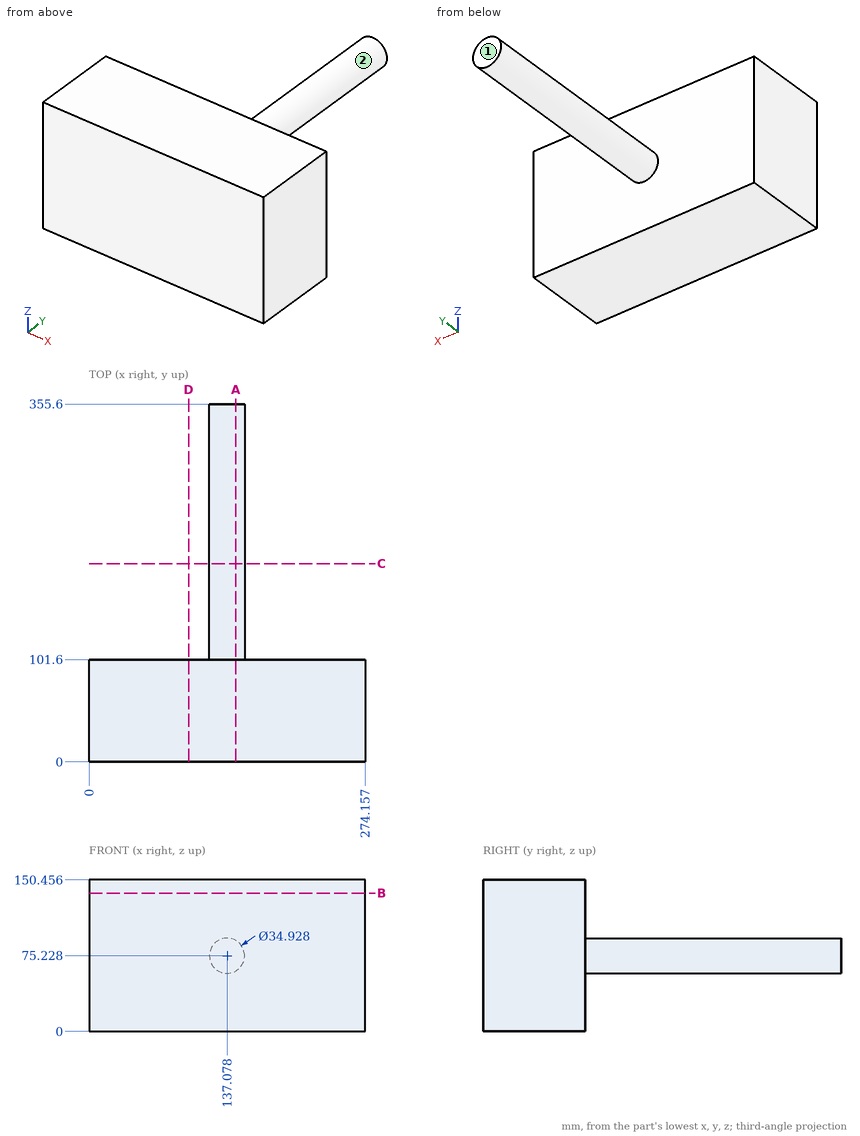
Print and shaded views of the part. All mm, measured from the part's lowest x, y and z. A direction names the side the tool comes from. Give positions to 0.01 mm unless a question says otherwise; leave off trailing zeros. Write each loop counter-clockwise with the first axis right and the second up, starting at its lowest first coordinate (ties: lowest second). Pieces come first, ordered by that corner, then holes. Notation, with made-up numbers: (43, 30) -> (72, 30) arc R16 ccw to (72, 50) -> close; hole circle Ø5 at (30, 46.5). An arc over 180 degrees is marked (long way). Use CSV: the item, a comma, the result in double quotes. Start each with the question number.
1) Cut at D-D on x = 99. List the corners of the cut face in (y, z) (1 decimal), plus the area to 3 significant figures.
2) Pin check, flat tips, straight feed: P1, Ø8, axis at y = 221.5, z = 93, coming from the -X side; P2, Ø5, axis at y = 204.5, z = 76, coming from the -X side (1 decimal). Stop position of each tip, or through.
3) Cut at B-B on z = 137.5. List the corners of the cut face in (x, y), plus the area to 3 significant figures.
4) Tool access for the marked faces 1 and 2: list every direction of +Z, -Z, +X, -X, +Y, -Y with a clear straight run to the whole face (end or side of a thin tool).
5) Drill centre lines: L1, parallel to Y at x = 113.5, z = 42.5; L2, parallel to Z at x = 143, y = 123.5; L3, parallel to X at y = 188, z = 87. Where is each one in solid material? Low to high.
6) Cut at A-A on x = 146. List the corners of the cut face in (y, z) (1 decimal).
7) Cut at C-C on y = 197. List the corners of the cut face in (x, z).
Final values:
1,outline,"(0, 0) -> (101.6, 0) -> (101.6, 150.5) -> (0, 150.5) -> close"
1,area,"15,300 mm2"
2,P1,"stops at x = 126.34"
2,P2,"stops at x = 119.6"
3,outline,"(0, 0) -> (274.16, 0) -> (274.16, 101.6) -> (0, 101.6) -> close"
3,area,"27,900 mm2"
4,face 1,"+Z, -Z, +X, -X, +Y"
4,face 2,"+Y"
5,L1,"y = 0 to 101.6"
5,L2,"z = 58.8 to 91.66"
5,L3,"x = 124.18 to 149.98"
6,outline,"(0, 0) -> (101.6, 0) -> (101.6, 60.2) -> (355.6, 60.2) -> (355.6, 90.2) -> (101.6, 90.2) -> (101.6, 150.5) -> (0, 150.5) -> close"
7,outline,"circle Ø34.93 at (137.08, 75.23)"
